Input: part model. Units: mm. Frame: model coordinates. Give positions to 0.01 mm unless a question says otherwise; leave off trailing zeros. Order: outer loops, then holes, each group sorted by start corner. A loop starts at its lowest first (then second) coordinate and runs counter-clockwise, first axis right, second up. Notation, with made-up numbers: (58, 13) - (71, 13) arc R35 cw to (71, 47) - close; hole circle Ø4 at (17.25, 69.5). An arc over 180 degrees is marked (long way). Answer in a Markdown table with one row per item. Add a question column.
from build123d import *

# Parameters (mm, degrees)
SKETCH1_R           = 2.5
SKETCH1_R_2         = 20
BOSS_EXTRUDE1_DEPTH = 5


with BuildPart() as part:
    # Sketch1 → Boss-Extrude1 (new body)
    with BuildSketch(Plane(origin=(0, 0, 0), x_dir=(1, 0, 0), z_dir=(0, 1, 0))):
        with BuildLine():
            Line((6, 0), (58.9, 0))
            ThreePointArc((58.9, 0), (63.142640687, 1.757359313), (64.9, 6))
            Line((64.9, 6), (64.9, 66))
            ThreePointArc((64.9, 66), (63.142640687, 70.242640687), (58.9, 72))
            Line((58.9, 72), (6, 72))
            ThreePointArc((6, 72), (1.757359313, 70.242640687), (0, 66))
            Line((0, 66), (0, 6))
            ThreePointArc((0, 6), (1.757359313, 1.757359313), (6, 0))
        make_face()
        with Locations((58.9, 66)):
            Circle(SKETCH1_R, mode=Mode.SUBTRACT)
        with Locations((58.9, 6)):
            Circle(SKETCH1_R, mode=Mode.SUBTRACT)
        with Locations((32.97, 36)):
            Circle(SKETCH1_R_2, mode=Mode.SUBTRACT)
        with BuildLine():
            Line((6, 3.5), (8, 3.5))
            ThreePointArc((8, 3.5), (10.5, 6), (8, 8.5))
            Line((8, 8.5), (6, 8.5))
            ThreePointArc((6, 8.5), (3.5, 6), (6, 3.5))
        make_face(mode=Mode.SUBTRACT)
        with BuildLine():
            Line((6, 63.5), (8, 63.5))
            ThreePointArc((8, 63.5), (10.5, 66), (8, 68.5))
            Line((8, 68.5), (6, 68.5))
            ThreePointArc((6, 68.5), (3.5, 66), (6, 63.5))
        make_face(mode=Mode.SUBTRACT)
    extrude(amount=BOSS_EXTRUDE1_DEPTH)


solid = part.part
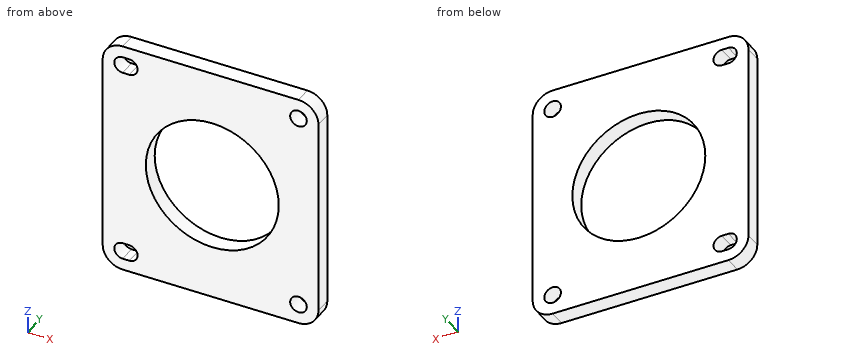
Q1. Section A-A, the plane x = 32.97. Return loops of the section in (y, z).
Q2. Line query: probe 1 along X at (y, z) = (3.15, -66); probe 2 along Z at (x, y) = (58.9, 1.25); probe 3 along X at (y, z) = (1.8, -36). Output: solid intervals per line, ascending.
Q3. Section B-B, the plane z = -49.5. Return loops of the section in (x, y), then the cut area to 3 significant figures.
Q4. Section C-C, the plane y = 1.9. Return loops of the section in (x, z).
Q5. Contact query for a flat-ended pin moving along its axis: P1, Ø4.5, axis at x = 58.9, z = -6, coming from the -Y side. Output: stop coordinate, or through.
Computed:
| question | item | result |
|---|---|---|
| 1 | outline | (0, -72) - (5, -72) - (5, -56) - (0, -56) - close; (0, -16) - (5, -16) - (5, 0) - (0, 0) - close |
| 2 | probe 1 | x = 0 to 3.5, 10.5 to 56.4, 61.4 to 64.9 |
| 2 | probe 2 | z = -72 to -68.5, -63.5 to -8.5, -3.5 to 0 |
| 2 | probe 3 | x = 0 to 12.97, 52.97 to 64.9 |
| 3 | outline | (0, 0) - (18.21, 0) - (18.21, 5) - (0, 5) - close; (47.73, 0) - (64.9, 0) - (64.9, 5) - (47.73, 5) - close |
| 3 | area | 177 mm^2 |
| 4 | outline | (0, -66) arc R6 ccw to (6, -72) - (58.9, -72) arc R6 ccw to (64.9, -66) - (64.9, -6) arc R6 ccw to (58.9, 0) - (6, 0) arc R6 ccw to (0, -6) - close; hole (6, -68.5) - (8, -68.5) arc R2.5 ccw to (8, -63.5) - (6, -63.5) arc R2.5 ccw to start; hole (6, -8.5) - (8, -8.5) arc R2.5 ccw to (8, -3.5) - (6, -3.5) arc R2.5 ccw to start; hole circle Ø40 at (32.97, -36); hole circle Ø5 at (58.9, -66); hole circle Ø5 at (58.9, -6) |
| 5 | P1 | passes through |
